Part print with two shaded views. Sizes in mm from the minimum x, y, z corner. A direction names the side the tool comes from. Round coordinates to 2 decimals unless told otherwise and drop trailing zeros. Write each loop counter-clockwise with the first axis right and the second up, starting at its lowest first coordinate (ties: lowest second). Pieces come first, ordered by that corner, then holes. Notation, with made-up numbers: (12, -39) -> (61, -39) arc R10 ccw to (61, -32) -> close; hole circle Ø9 at (-4, 31). An arc over 180 degrees is marked (long way). Return JSON: item names as keys, results as strings.
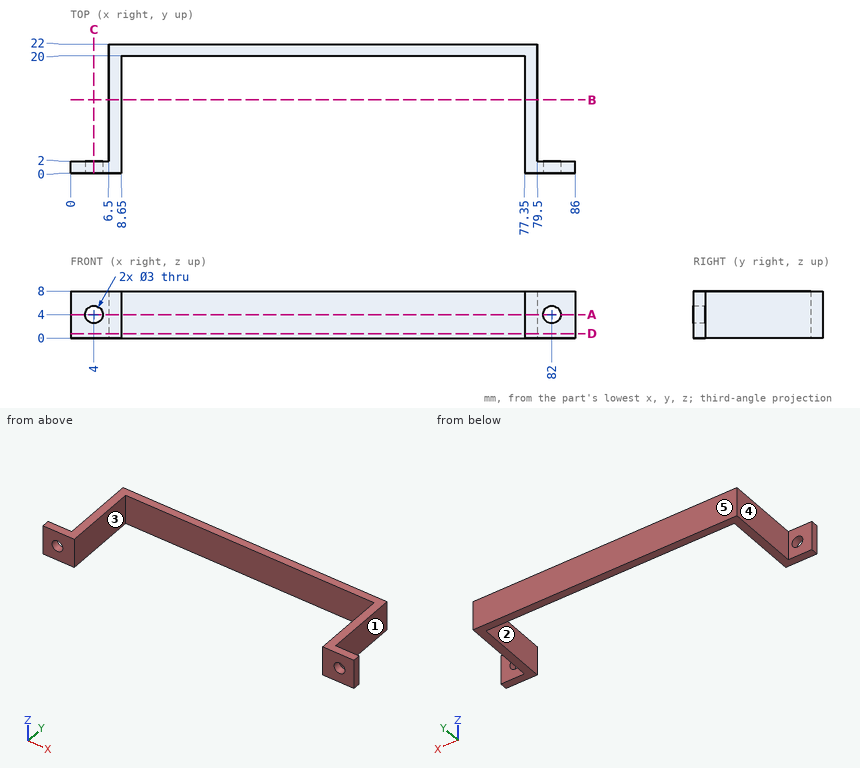
Q1. Two-plate mould, pull along X, no slides. Class the marked faces 3, 4 and 5: +X half, -X half, draft (parallel to the pull), parting line (faces both ways), or undercut.
Verdict:
{"face 3": "undercut", "face 4": "-X half", "face 5": "draft"}
Q2. Saw through at B-B on y = 12.5. List the corners of the cut face in (x, z).
Verdict:
{"outline": "(6.5, 0) -> (8.65, 0) -> (8.65, 8) -> (6.5, 8) -> close; (77.35, 0) -> (79.5, 0) -> (79.5, 8) -> (77.35, 8) -> close"}
Q3. Saw through at A-A on z = 4. List the corners of the cut face in (x, y), then the cut area to 3 significant figures.
Verdict:
{"outline": "(0, 0) -> (2.5, 0) -> (2.5, 2) -> (0, 2) -> close; (5.5, 0) -> (8.65, 0) -> (8.65, 20) -> (77.35, 20) -> (77.35, 0) -> (80.5, 0) -> (80.5, 2) -> (79.5, 2) -> (79.5, 22) -> (6.5, 22) -> (6.5, 2) -> (5.5, 2) -> close; (83.5, 0) -> (86, 0) -> (86, 2) -> (83.5, 2) -> close", "area": "246 mm²"}
Q4. 3-axis set-ups, long thin cutter, end or side, ignore diameter. For the marked faces 1 and 2: which of +Z, -Z, +X, -X, +Y, -Y reach the whole face in a straight line?
Verdict:
{"face 1": "+Z, -Z, +X, +Y", "face 2": "+Z, -Z, -Y"}
Q5. Pin check, flat tips, straight feed: pin 1 Ø4 at (y, z) = (12.5, 2.5) entering from -X; pin 2 Ø3.5 at (x, z) = (4, 4) entering from +Y; pin 3 Ø1.5 at (x, y) = (11, 11) entering from -Z; pin 4 Ø2.5 at (x, z) = (38, 4.5) entering from -Y. Stop position of each tip, or through.
Verdict:
{"pin 1": "stops at x = 6.5", "pin 2": "stops at y = 2", "pin 3": "passes through", "pin 4": "stops at y = 20"}
Q6. Saw through at D-D on z = 0.75. List the corners of the cut face in (x, y).
Verdict:
{"outline": "(0, 0) -> (8.65, 0) -> (8.65, 20) -> (77.35, 20) -> (77.35, 0) -> (86, 0) -> (86, 2) -> (79.5, 2) -> (79.5, 22) -> (6.5, 22) -> (6.5, 2) -> (0, 2) -> close"}
Q7. Wall check: L1, parallel to X at y = 0.8, z = 4; L2, parallel to X at y = 19.25, z = 6.75; L3, parallel to Y at x = 66, z = 3.75. Give the ranges that are in metal, low to high.
Verdict:
{"L1": "x = 0 to 2.5, 5.5 to 8.65, 77.35 to 80.5, 83.5 to 86", "L2": "x = 6.5 to 8.65, 77.35 to 79.5", "L3": "y = 20 to 22"}
Q8. Saw through at C-C on x = 4. List the corners of the cut face in (y, z).
Verdict:
{"outline": "(0, 0) -> (2, 0) -> (2, 2.5) -> (0, 2.5) -> close; (0, 5.5) -> (2, 5.5) -> (2, 8) -> (0, 8) -> close"}
